Geometry check sheet. Reference: the model listing, model coordinates, mm. A direction names the side the tool comes from. Coordinates: 2 decimals unless noted, no trailing zeros. Write each loop counter-clockwise with the first axis right and the second up, starting at its lowest first coordinate (ties: lowest second). Pieces come first, ordered by that corner, then holes. Notation, with made-up numbers: M 33.5,-15 L 88.5,-15 A24 ccw 88.5,16 Z; hole C 59,-23.75 d8. An arc over 180 degrees is marked long. Put each result on its own line as item: value. Start each with the question number.
1) Mould release check, pull along Y, two halves, no side actions. Record for faces 4 (the flat face through (7, 1, 2.31)), 5 (the flat face through (5.2, 0.2, 3.91)): released by +Y, released by -Y, zero draft, split by the parting line, or undercut.
2) Gauge pin test, flat ends, axial feed: pin 1 (2 mm diameter, centred on x = 2, z = 18.5, fed in from +Y); pin 2 (4 mm diameter, centred on x = 1, z = 11, fed in from -Y); pin 3 (1.8 mm diameter, centred on x = -1.5, y = 0.5, fed in from +Z). Record the tip position at first contact, or that the pin passes through.
3) Cross-section at A-A on z = 9.5. Record the cut outline in (x, y), plus the area to 3 significant figures.
4) Cross-section at B-B on x = -8. Record the cut outline in (y, z).
5) Scan lines: line 1 along Y through (x, z) = (0, 1.4); line 2 along X through (y, z) = (-0.75, 3.25); line 3 along Z through (x, y) = (-7.5, 4.75). Record each from-to range of solid material in increasing order.
6) Set-up check for faces 1 (the cylindrical face through (-5.56, -0.54, 3.12)), 2 (the flat face through (-3, 3, 0)), 3 (the flat face through (0, 0, 1.91)): record each of +Z, -Z, +X, -X, +Y, -Y from which the full face is reachable in a straight line by a thin tool's end or side.
from build123d import *

# Parameters (mm, degrees)
ESQUISSE1_R                                        = 12
BOSS_EXTRU_1_DEPTH                                 = 3.91
ESQUISSE6_R                                        = 4
ENL_V_MAT_EXTRU_2_DEPTH                            = 1.91
BOSS_EXTRU_2_DEPTH                                 = 20
CHAMBRAGE_POUR_VIS_T_TE_RONDE_BOMB_E_M_D           = 2.4
CHAMBRAGE_POUR_VIS_T_TE_RONDE_BOMB_E_M_CBORE_D     = 5
CHAMBRAGE_POUR_VIS_T_TE_RONDE_BOMB_E_M_CBORE_DEPTH = 1.6
R_P_TITION_CIRCULAIRE2_COUNT                       = 4


with BuildPart() as part:
    # Esquisse1 → Boss.-Extru.1 (new body)
    with BuildSketch(Plane.XY):
        Circle(ESQUISSE1_R)
    extrude(amount=BOSS_EXTRU_1_DEPTH)

    # Esquisse6 → Enlèv. mat.-Extru.2 (cut)
    with BuildSketch(Plane(origin=(0, 0, 0), x_dir=(-1, 0, 0), z_dir=(0, 0, -1))):
        Circle(ESQUISSE6_R)
    extrude(amount=-ENL_V_MAT_EXTRU_2_DEPTH, mode=Mode.SUBTRACT)

    # Esquisse7 → Boss.-Extru.2 (add)
    # profile 1 of 2: a face of its own
    with BuildSketch(Plane.XY.offset(3.91)):
        with BuildLine():
            Line((-3.716127016, -3.27), (0, -3.27))
            Line((0, -3.27), (3.716127016, -3.27))
            ThreePointArc((3.716127016, -3.27), (4.631270276, -1.747522714), (4.95, 0))
            ThreePointArc((4.95, 0), (-1.747522714, 4.631270276), (-3.716127016, -3.27))
        make_face()
        with BuildLine():
            Line((-1.956655309, 2.62), (1.956655309, 2.62))
            ThreePointArc((1.956655309, 2.62), (3.103248298, -1.030897667), (0, -3.27))
            ThreePointArc((0, -3.27), (-3.103248298, -1.030897667), (-1.956655309, 2.62))
        make_face(mode=Mode.SUBTRACT)
    # profile 2 of 2: a face of its own
    with BuildSketch(Plane.XY.offset(3.91)):
        with BuildLine():
            Line((3.716127016, -3.27), (0, -3.27))
            Line((0, -3.27), (-3.716127016, -3.27))
            ThreePointArc((-3.716127016, -3.27), (0, -4.95), (3.716127016, -3.27))
        make_face()
    extrude(amount=BOSS_EXTRU_2_DEPTH)

    # Chambrage pour vis à tête ronde bombée M21 (through all)
    with Locations(Plane.XY.offset(3.91)):
        with Locations((0, 8)):
            chambrage_pour_vis_t_te_ronde_bomb_e_m = CounterBoreHole(CHAMBRAGE_POUR_VIS_T_TE_RONDE_BOMB_E_M_D / 2, CHAMBRAGE_POUR_VIS_T_TE_RONDE_BOMB_E_M_CBORE_D / 2, CHAMBRAGE_POUR_VIS_T_TE_RONDE_BOMB_E_M_CBORE_DEPTH)

    # Répétition circulaire2: Chambrage pour vis à tête ronde bombée M21 ×4 about axis
    r_p_tition_circulaire2_axis = Axis((0, 0, 0), (0, 0, 1))
    for i in range(1, R_P_TITION_CIRCULAIRE2_COUNT):
        add(chambrage_pour_vis_t_te_ronde_bomb_e_m.rotate(r_p_tition_circulaire2_axis, i * 360 / R_P_TITION_CIRCULAIRE2_COUNT), mode=Mode.SUBTRACT)


solid = part.part
Answer key:
1. face 4: undercut
1. face 5: zero draft
2. pin 1: stops at y = 4.85
2. pin 2: stops at y = -4.95
2. pin 3: stops at z = 3.91
3. outline: C 0,0 d9.9; hole M -1.96,2.62 A3.27 ccw long 1.96,2.62 Z
3. area: 45.1 mm²
4. outline: M -8.94,0 L -1.2,0 L -1.2,2.31 L -2.5,2.31 L -2.5,3.91 L -8.94,3.91 Z; M 1.2,0 L 8.94,0 L 8.94,3.91 L 2.5,3.91 L 2.5,2.31 L 1.2,2.31 Z
5. line 1: y = -12 to -9.2, -6.8 to -4, 4 to 6.8, 9.2 to 12
5. line 2: x = -11.98 to -10.38, -5.62 to 5.62, 10.38 to 11.98
5. line 3: z = 0 to 3.91
6. face 1: +Z
6. face 2: -Z, +X, -X, +Y, -Y
6. face 3: -Z
